```python
from build123d import *

# Parameters (mm, degrees)
SKETCH1_R               = 3.175
BOSS_EXTRUDE1_DEPTH     = 50.8
CHAMFER1_SIZE           = 0.254
SKETCH2_R               = 0.8001
CUT_EXTRUDE1_DEPTH      = 4.175
CUT_EXTRUDE1_DEPTH_BACK = 4.175


with BuildPart() as part:
    # Sketch1 → Boss-Extrude1 (new body)
    with BuildSketch(Plane(origin=(0, 0, 0), x_dir=(0, 0, -1), z_dir=(1, 0, 0))):
        Circle(SKETCH1_R)
    extrude(amount=-BOSS_EXTRUDE1_DEPTH)

    # Chamfer1
    chamfer1_edges = [part.edges().sort_by_distance(p)[0] for p in [
        (0, 0, 3.175),
        (-50.8, 0, 3.175),
    ]]
    chamfer(chamfer1_edges, length=CHAMFER1_SIZE)

    # Sketch2 → Cut-Extrude1 (cut, two sides)
    with BuildSketch(Plane(origin=(0, 0, 0), x_dir=(1, 0, 0), z_dir=(0, 1, 0))) as cut_extrude1_sk:
        with Locations((-15.875, 0)):
            Circle(SKETCH2_R)
    extrude(amount=CUT_EXTRUDE1_DEPTH, mode=Mode.SUBTRACT)
    extrude(cut_extrude1_sk.sketch, amount=-CUT_EXTRUDE1_DEPTH_BACK, mode=Mode.SUBTRACT)


solid = part.part
```
Can you work these out from the model? Positions are in its coordinate system, mm. Coordinates: 2 decimals unless noted, no trailing zeros. Write each loop counter-clockwise with the first axis right and the second up, starting at its lowest first coordinate (ties: lowest second). Pieces come first, ordered by that corner, then holes. Notation, with made-up numbers: (-37.75, 65) - (19.25, 65) arc R20 ccw to (19.25, 94) - close; hole circle Ø6 at (47.25, 1.5). An arc over 180 degrees is marked (long way). Return JSON: item names as keys, results as strings.
Q1. If we section it at B-B (x = -38): Please give me the cut outline in (y, z) (3 decimals), then the cut area to 3 significant figures.
Computed values:
{"outline": "circle Ø6.35 at (0, 0)", "area": "31.7 mm2"}
Q2. If we section it at A-A (z = 0): Please give me the cut outline in (x, y) (3 decimals).
Computed values:
{"outline": "(-50.8, -2.921) - (-50.546, -3.175) - (-16.675, -3.175) - (-16.675, 3.175) - (-50.546, 3.175) - (-50.8, 2.921) - close; (-15.075, -3.175) - (-0.254, -3.175) - (0, -2.921) - (0, 2.921) - (-0.254, 3.175) - (-15.075, 3.175) - close"}
Q3. Please list where these lines run through material, in increasing order: L1, parallel to X at y = -0.8, z = 0; L2, parallel to Y at x = -6, z = 1.25; L3, parallel to Z at x = -27.5, y = 0.25. Write a range as from..to.
Computed values:
{"L1": "x = -50.8..-16.68, -15.07..0", "L2": "y = -2.92..2.92", "L3": "z = -3.17..3.17"}
Q4. I'm going to push a flat-ended pin straight in: pin 1 Ø3 at (x, y) = (-44, -2) entering from -Z. Where does the tip first touch, or does it pass through?
Computed values:
{"pin 1": "stops at z = -3.14"}
